Geometry: final body of the model. Coordinates: model frame, mm. A direction names the side the tool comes from. Give positions to 0.01 mm unless a question says otherwise; leave off trailing zeros. Order: outer loops, then holes, each group sorted by start corner. A loop starts at its lowest first (then second) coordinate and runs counter-clockwise, first axis right, second up. Notation, with made-up numbers: M 19,19 L 46,19 A19 ccw 46,53 Z; hole C -38,81 d8. An arc over 180 degrees is marked long. One line per item, written item: value. Start each with the question number.
```python
from build123d import *

# Parameters (mm, degrees)
F0_W     = 12
F0_H     = 12
F1_DEPTH = 30
F2_DEPTH = 12
F3_R     = 4.15
F4_DEPTH = 45


with BuildPart() as f1:
    # F0 (on Top) → F1 (new body)
    with BuildSketch(Plane.XY):
        Rectangle(F0_W, F0_H)
    extrude(amount=F1_DEPTH)

    # F0 (on Top) → F2 (join)
    with BuildSketch(Plane.XY):
        with Locations((-12, 0)):
            Rectangle(F0_W, F0_H)
        with Locations((12, 0)):
            Rectangle(F0_W, F0_H)
    extrude(amount=F2_DEPTH)

    # F3 (on face) → F4 (cut)
    with BuildSketch(Plane.YZ.offset(18)):
        with Locations((0, 6.070589)):
            Circle(F3_R)
    extrude(amount=-F4_DEPTH, mode=Mode.SUBTRACT)


solid = f1.part
```
Q1. Section query B-B on z = 7.75. Return loops of the section in (x, y) (3 decimals), and give its area (3 significant figures).
Q2. Section query D-D on y = 2.75. Return loops of the section in (x, z), and give its area (3 significant figures).
Q3. Set-up query: faces 1 (the face through (0, 0, 30)), 2 (the face through (-12, 0, 12)), 3 (the face through (6, 0, 21)). Return all of +Z, -Z, +X, -X, +Y, -Y with unobstructed straight access to the full face (end or side cutting, diameter ignored); none if empty.
Q4. Section query A-A on y = 0. Return loops of the section in (x, z).
Q5. Ray query, line 1 along Z through (x, y) = (5, 0); line 2 along Z through (x, y) = (7, 0); line 3 along X through (y, z) = (-2.75, 12.25). Return the intervals inside material, ascending. Write a range as [from, to].
Q6. Section query C-C on x = 14. Return loops of the section in (y, z).
Q7. Mould query, pull axis Z, two halves, no side actions, for faces 4 (the face through (-6, 0, 21)), 5 (the face through (0, 0, 0)), 6 (the face through (12, 0, 12)), 7 (the face through (0.25, 2.23, 9.57)). Classes: +Z half, -Z half, draft (parallel to the pull), parting line (faces both ways), or undercut.
Q8. Contact query for flat-ended pins moving along their axis: pin 1 (5 mm diameter, centred on y = 0, z = 6.07, fed in from -X); pin 2 (6 mm diameter, centred on y = -1.5, z = 21, fed in from +X); pin 3 (6 mm diameter, centred on x = -12, y = 2.5, fed in from +Z); pin 4 (1 mm diameter, centred on y = -2.5, z = 25.5, fed in from -X). Output: stop coordinate, or through.
Results below:
1. outline: M -18,-6 L 18,-6 L 18,-3.795 L -18,-3.795 Z; M -18,3.795 L 18,3.795 L 18,6 L -18,6 Z
1. area: 159 mm2
2. outline: M -18,0 L 18,0 L 18,2.96 L -18,2.96 Z; M -18,9.18 L 18,9.18 L 18,12 L 6,12 L 6,30 L -6,30 L -6,12 L -18,12 Z
2. area: 424 mm2
3. face 1: +Z, +X, -X, +Y, -Y
3. face 2: +Z, -X, +Y, -Y
3. face 3: +Z, +X, +Y, -Y
4. outline: M -18,0 L 18,0 L 18,1.92 L -18,1.92 Z; M -18,10.22 L 18,10.22 L 18,12 L 6,12 L 6,30 L -6,30 L -6,12 L -18,12 Z
5. line 1: [0, 1.92], [10.22, 30]
5. line 2: [0, 1.92], [10.22, 12]
5. line 3: [-6, 6]
6. outline: M -6,0 L 6,0 L 6,12 L -6,12 Z; hole C 0,6.07 d8.3
7. face 4: draft
7. face 5: -Z half
7. face 6: +Z half
7. face 7: undercut
8. pin 1: through
8. pin 2: x = 6
8. pin 3: z = 12
8. pin 4: x = -6
